```python
from build123d import *

# Parameters (mm, degrees)
SKETCH_R        = 12.47775
PAD_DEPTH       = 18.7833
SKETCH001_R     = 3.44805
PAD001_DEPTH    = 2.667
SKETCH002_R     = 1.9939
PAD002_DEPTH    = 9.652
SKETCH003_W     = 1.605508
SKETCH003_H     = 4.122735
POCKET_DEPTH    = 8.0645
SKETCH004_R     = 1.27
POCKET001_DEPTH = 6.35
SKETCH005_R     = 11.938
PAD003_DEPTH    = 30.5689
SKETCH006_R     = 4.191
PAD004_DEPTH    = 2.0447
SKETCH007_W     = 0.3175
SKETCH007_H     = 3.0099
PAD005_DEPTH    = 5.5118
SKETCH008_R     = 0.9779
PAD006_DEPTH    = 1.0541


with BuildPart() as part:
    # Sketch → Pad (new body)
    with BuildSketch(Plane.XY):
        Circle(SKETCH_R)
    extrude(amount=-PAD_DEPTH)

    # Sketch001 → Pad001 (new body)
    with BuildSketch(Plane.XY):
        Circle(SKETCH001_R)
    extrude(amount=PAD001_DEPTH)

    # Sketch002 → Pad002 (new body)
    with BuildSketch(Plane.XY.offset(2.667)):
        Circle(SKETCH002_R)
    extrude(amount=PAD002_DEPTH)

    # Sketch003 → Pocket (cut)
    with BuildSketch(Plane.XY.offset(12.319)):
        with Locations((1.437754, -0.02757)):
            Rectangle(SKETCH003_W, SKETCH003_H)
    extrude(amount=-POCKET_DEPTH, mode=Mode.SUBTRACT)

    # Sketch004 → Pocket001 (cut)
    with BuildSketch(Plane.XY):
        with Locations((8.46455, 0)):
            Circle(SKETCH004_R)
        with Locations((-8.46455, 0)):
            Circle(SKETCH004_R)
    extrude(amount=-POCKET001_DEPTH, mode=Mode.SUBTRACT)

    # Sketch005 → Pad003 (new body)
    with BuildSketch(Plane(origin=(0, 0, -18.7833), x_dir=(1, 0, 0), z_dir=(0, 0, -1))):
        Circle(SKETCH005_R)
    extrude(amount=PAD003_DEPTH)

    # Sketch006 → Pad004 (new body)
    with BuildSketch(Plane(origin=(0, 0, -49.3522), x_dir=(1, 0, 0), z_dir=(0, 0, -1))):
        Circle(SKETCH006_R)
    extrude(amount=PAD004_DEPTH)

    # Sketch007 → Pad005 (new body)
    with BuildSketch(Plane(origin=(0, 0, -49.3522), x_dir=(1, 0, 0), z_dir=(0, 0, -1))):
        with Locations((9.3599, 0)):
            Rectangle(SKETCH007_W, SKETCH007_H)
        with Locations((-7.9629, 0.00127)):
            Rectangle(SKETCH007_W, SKETCH007_H)
    extrude(amount=PAD005_DEPTH)

    # Sketch008 → Pad006 (new body)
    with BuildSketch(Plane(origin=(0, 0, -51.3969), x_dir=(1, 0, 0), z_dir=(0, 0, -1))):
        Circle(SKETCH008_R)
    extrude(amount=PAD006_DEPTH)


solid = part.part
```
Can you work these out from the model? Positions are in its coordinate system, mm. A direction names the side the tool comes from. Give positions to 0.01 mm unless a question says otherwise; leave off trailing zeros. Loops run counter-clockwise (first coordinate to the right, second up) from the corner with the lowest first, then second, coordinate; pieces in that order, holes last. Notation, with made-up numbers: M 78.5,-31.5 L 105.5,-31.5 A27 ccw 105.5,0.5 Z; hole C 3.25,13 d4. An arc over 180 degrees is marked long. Use one line per item in the form item = value. Start each with the question number.
(1) I want a section at B-B, the plane z = -30. Write out the boundary of the cut face in (x, y).
(2) Please list where these lines run through material, in increasing order: line 1 (Z direction, x = -7.5, y = 5.5); line 2 (X direction, y = 0.5, z = -43.5); line 3 (Y direction, x = -2, z = -16).
(3) Thinking about a two-plate mould opening in Y: for faces 4 (the flat face through (0, 0, -52.451)), 5 (the flat face through (8, 0, -6.35)), 6 (the flat face through (-8, 0, -6.35)), 7 (the cylindrical face through (-1.99, 0.09, 6.35)), which applies, released by +Y, released by -Y, zero draft, split by the parting line, or undercut?
(4) I'm going to push flat-ended pins straight in: P1, Ø10, axis at x = 2, y = 3.5, coming from the -Z side; P2, Ø3, axis at x = -9, y = 0.5, coming from the +Z side; P3, Ø7, axis at x = -4, y = -4, coming from the -Z side; P4, Ø4, axis at y = 9, z = 2.5, coming from the +X side. Where does each tip first touch, or does it pass through?
(5) I want a section at A-A, the plane x = 0. Write out the boundary of the cut face in (y, z), and give its area (3 significant figures).
(6) I want a section at C-C, the plane y = -9.75. Write out the boundary of the cut face in (x, z), and give its area (3 significant figures).
(7) On a 3-axis mill with a long thin cutter (end or side, diameter ignored), from which of +Z, -Z, +X, -X, +Y, -Y can I reach the whole of each face in a straight line? I mean faces 1 (the flat face through (-8.122, 0, -52)), 2 (the cylindrical face through (-2.588, 11.654, -33.854)), 3 (the flat face through (3, -3, 0)). Say none if no direction works.
(8) I want a section at D-D, the plane x = 6. Write out the boundary of the cut face in (y, z), and give its area (3 significant figures).
Worked out:
q1.outline = C 0,0 d23.88
q2.line_1 = -49.35 to 0
q2.line_2 = -11.93 to 11.93
q2.line_3 = -12.32 to 12.32
q3.face_4 = zero draft
q3.face_5 = undercut
q3.face_6 = undercut
q3.face_7 = split by the parting line
q4.P1 = -52.45
q4.P2 = 0
q4.P3 = -51.4
q4.P4 = through
q5.outline = M -12.48,-18.78 L -11.94,-18.78 L -11.94,-49.35 L -4.19,-49.35 L -4.19,-51.4 L -0.98,-51.4 L -0.98,-52.45 L 0.98,-52.45 L 0.98,-51.4 L 4.19,-51.4 L 4.19,-49.35 L 11.94,-49.35 L 11.94,-18.78 L 12.48,-18.78 L 12.48,0 L 3.45,0 L 3.45,2.67 L 1.99,2.67 L 1.99,12.32 L -1.99,12.32 L -1.99,2.67 L -3.45,2.67 L -3.45,0 L -12.48,0 Z
q5.area = 1,270 mm²
q6.outline = M -7.79,-18.78 L -6.89,-18.78 L -6.89,-49.35 L 6.89,-49.35 L 6.89,-18.78 L 7.79,-18.78 L 7.79,0 L -7.79,0 Z
q6.area = 714 mm²
q7.face_1 = -Z, -X, +Y, -Y
q7.face_2 = -Z
q7.face_3 = +Z
q8.outline = M -10.94,-18.78 L -10.32,-18.78 L -10.32,-49.35 L 10.32,-49.35 L 10.32,-18.78 L 10.94,-18.78 L 10.94,0 L -10.94,0 Z
q8.area = 1,040 mm²
